Check sheet for the modelled part. Datum: model origin and axes. Units: mm. Face numbers are marked on the shaded views. A direction names the side the tool comes from. Give positions to 0.01 mm unless a question says otherwise; leave off trailing zeros. Loops run counter-clockwise (first coordinate to the right, second up) from the corner with the lowest first, then second, coordinate; pieces in that order, holes last. Notation, with made-up numbers: (44, 13) -> (56, 13) arc R32 cw to (56, 47) -> close; hole circle Ø5 at (65.25, 87). An arc over 180 degrees is marked (long way). Answer as CSV lines item,"result". Start each with the question number.
(1) Gauge pin test, flat end, axial feed: pin 1 Ø1 at (y, z) = (1.5, 1.5) entering from +X. Record the tip position at first contact, or that the pin passes through.
(2) Access from +Z, -Z, +X, -X, +Y, -Y to the whole of each face (thin tool, end or side, straight path). Record for the marked faces 1, 2 and 3.
(3) Release check for a two-part mould opening along Y. For the marked faces 4, 5, 6 and 7 record: pulls with the +Y half, pulls with the -Y half, needs draft (parallel to the pull), parting line crosses it, or undercut.
(4) Section check B-B on y = 2.5. Enter the section's corners in (x, z).
(5) Material ranges on line 1 (X direction, y = 2.5, z = 0.4); line 2 (X direction, y = 0.75, z = 1.35); line 3 (Y direction, x = -2.5, z = 0.3), recorded low to high. Write a range as from..to.
(6) Section check A-A on x = 0. Enter the section's corners in (y, z) (3 decimals), plus the area to 3 significant figures.
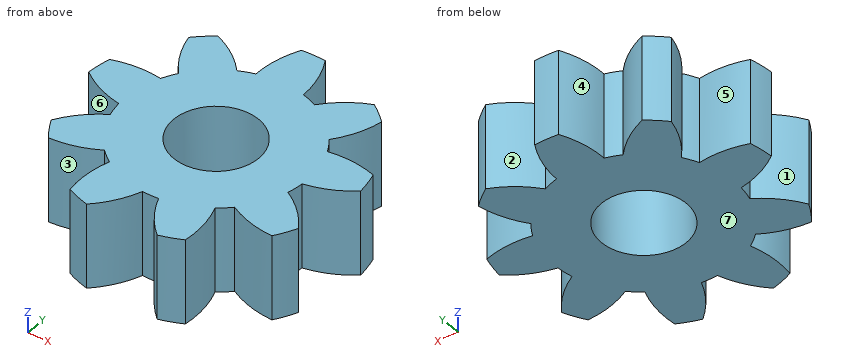
Autodesk Inventor part; units mm, degrees
ref_plane "Work Plane2" through (0, 0, 1) normal (0, 0, 1) x (1, 0, 0)
ref_plane "Work Plane8" through (0, 0, 0) normal (0.9396926, 0.3420201, 0) x (0, 0, 1)
ref_plane "Work Plane9" through (0, 0, 0) normal (1, 0, 0) x (0, 1, 0)
sketch "Sketch1" plane through (0, 0, 0) normal (0, 0, 1) x (1, 0, 0)
  circle A0 centre (0, 0) radius 3.1526
  dimension "d0" = 6.3051
extrude "Extrusion1" add sketch "Sketch1" along normal blind 2
ref_plane "Work Plane2" through (0, 0, 1) normal (0, 0, 1) x (1, 0, 0)
sketch "Sketch2" plane through (0, 0, 0) normal (0, 0, -1) x (-1, 0, 0)
  circle A0 centre (0, 0) radius 3.1526
  circle A1 centre (0, 0) radius 2.25
  dimension "d3" = 4.5
surface extrude "Pitch Diameter" sketch "Sketch2" against normal through all shown no curves A1
ref_plane "Work Plane8" through (0, 0, 0) normal (0.9396926, 0.3420201, 0) x (0, 0, 1)
ref_plane "Work Plane9" through (0, 0, 0) normal (1, 0, 0) x (0, 1, 0)
spur gear teeth "Spur Gear" teeth 9 pitch diameter 4.5 tip diameter 6.3051 root diameter 4.25 face width 2 start plane through (0, 0, 0) normal (0, 0, -1) x (-1, 0, 0)
sketch "Sketch3" plane through (0, 0, 2) normal (0, 0, 1) x (1, 0, 0)
  circle A0 centre (0, 0) radius 1
  dimension "d49" = 2
extrude "Extrusion2" cut sketch "Sketch3" against normal up to surface (2 mm away)
equation "\"d0\" = da_da"
equation "\"d1\" = da_b"
equation "\"d3\" = da_d"
equation "\"d16\" = da_aw"
equation "\"d43\" = da_aw"
equation "\"d46\" = da_aw"
properties part number "Spur Gear2" material "Steel"
Working result:
1,pin 1,"stops at x = 2.17"
2,face 1,"+Z, -Z, -X"
2,face 2,"+Z, -Z, +Y"
2,face 3,"+Z, -Z, -Y"
3,face 4,"pulls with the +Y half"
3,face 5,"undercut"
3,face 6,"undercut"
3,face 7,"needs draft"
4,outline,"(-1.92, 0) -> (-1.63, 0) -> (-1.63, 2) -> (-1.92, 2) -> close; (-0.5, 0) -> (0.5, 0) -> (0.5, 2) -> (-0.5, 2) -> close; (1.63, 0) -> (1.92, 0) -> (1.92, 2) -> (1.63, 2) -> close"
5,line 1,"x = -1.92..-1.63, -0.5..0.5, 1.63..1.92"
5,line 2,"x = -3.06..-0.66, 0.66..3.06"
5,line 3,"y = -1.8..-0.89, -0.08..0.92"
6,outline,"(-2.125, 0) -> (-1, 0) -> (-1, 2) -> (-2.125, 2) -> close; (1, 0) -> (3.153, 0) -> (3.153, 2) -> (1, 2) -> close"
6,area,"6.56 mm^2"
